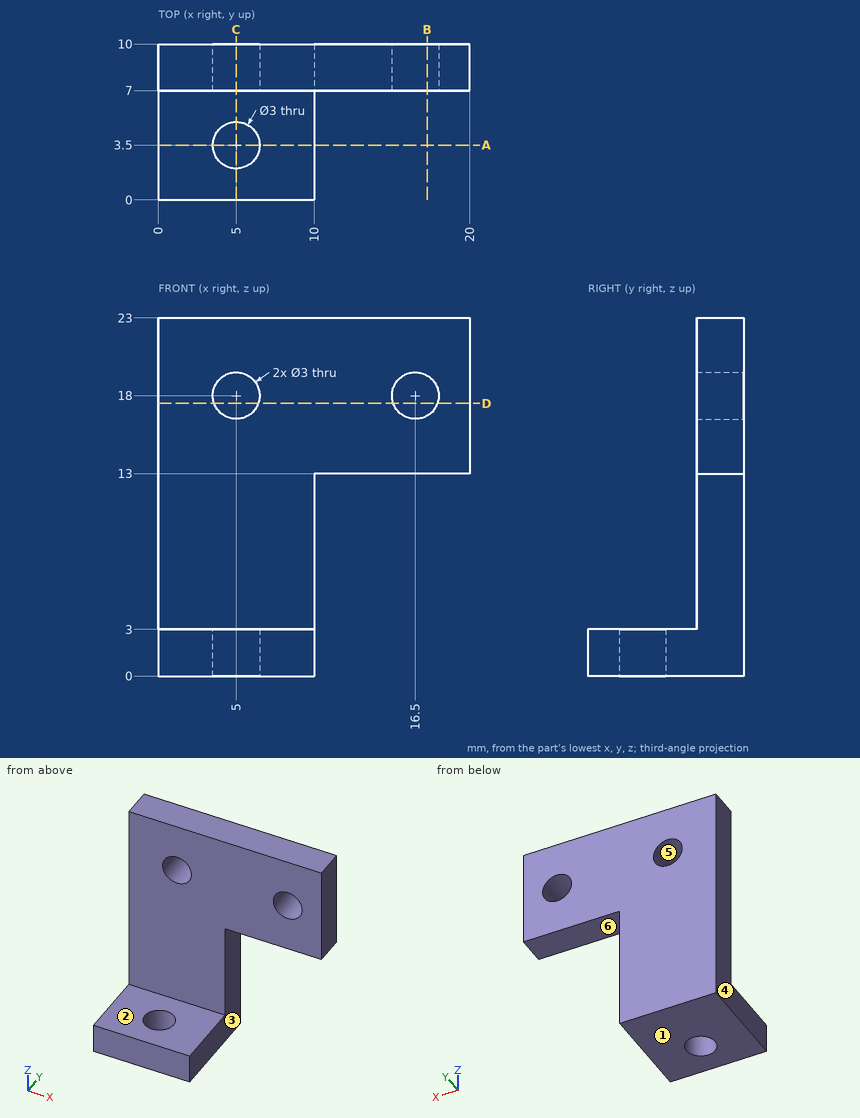
Can you work these out from the drawing? Everything is in mm from the part's minimum corner. A direction names the side the tool comes from. Coordinates: 2 decimals unless noted, no trailing zeros. Loops run counter-clockwise (first coordinate to the right, second up) from the corner with the lowest first, then second, coordinate; pieces in that order, holes last. Notation, with made-up numbers: (43, -30.5) -> (96, -30.5) arc R34 ccw to (96, 3.5) -> close; hole circle Ø3 at (26.5, 15). An arc over 180 degrees is marked (long way). Return JSON: item names as keys, results as strings.
1) If we section it at D-D, the plane z = 17.5: Write out the boundary of the cut face in (x, y).
Results below:
{"outline": "(0, 7) -> (3.59, 7) -> (3.59, 10) -> (0, 10) -> close; (6.41, 7) -> (15.09, 7) -> (15.09, 10) -> (6.41, 10) -> close; (17.91, 7) -> (20, 7) -> (20, 10) -> (17.91, 10) -> close"}
2) Thinking about a two-plate mould opening in Z: for the marked faces 4, 5 and 6, which applies, +Z half, -Z half, draft (parallel to the pull), parting line (faces both ways), or undercut?
Results below:
{"face 4": "draft", "face 5": "undercut", "face 6": "-Z half"}
3) For the marked faces 1, 2 and 3, which set-ups out of +Z, -Z, +X, -X, +Y, -Y let a thin tool reach every point of the face, with its end or its side?
Results below:
{"face 1": "-Z, +X, -X, +Y, -Y", "face 2": "+Z, +X, -X, -Y", "face 3": "-Z, +X, +Y, -Y"}
4) If we section it at A-A, the plane y = 3.5: Write out the boundary of the cut face in (x, z), then the cut area to 3 significant figures.
Results below:
{"outline": "(0, 0) -> (3.5, 0) -> (3.5, 3) -> (0, 3) -> close; (6.5, 0) -> (10, 0) -> (10, 3) -> (6.5, 3) -> close", "area": "21.0 mm²"}
5) Will these pins go through, and if not, where does the flat tip stop? pin 1 (5 mm diameter, centred on x = 6.5, y = 4, fed in from +Z); pin 2 (0.9 mm diameter, centred on x = 13, y = 9, fed in from -Z); pin 3 (4 mm diameter, centred on y = 4.5, z = 6, fed in from -X); pin 4 (8 mm diameter, centred on x = 3.5, z = 18, fed in from -Y).
Results below:
{"pin 1": "z = 3", "pin 2": "z = 13", "pin 3": "through", "pin 4": "y = 7"}
6) If we section it at B-B, the plane x = 17.25: Write out the boundary of the cut face in (y, z).
Results below:
{"outline": "(7, 13) -> (10, 13) -> (10, 16.7) -> (7, 16.7) -> close; (7, 19.3) -> (10, 19.3) -> (10, 23) -> (7, 23) -> close"}
7) If we section it at C-C, the plane x = 5: Write out the boundary of the cut face in (y, z).
Results below:
{"outline": "(0, 0) -> (2, 0) -> (2, 3) -> (0, 3) -> close; (5, 0) -> (10, 0) -> (10, 16.5) -> (7, 16.5) -> (7, 3) -> (5, 3) -> close; (7, 19.5) -> (10, 19.5) -> (10, 23) -> (7, 23) -> close"}
8) I need wall thicknesses on line 1 (X direction, y = 8, z = 18); line 2 (Y direction, x = 5, z = 1.6); line 3 (Y direction, x = 12.25, z = 14.75). Which ranges of each line are inside material? Lowest first, please. Write a range as from..to.
Results below:
{"line 1": "0..3.5, 6.5..15, 18..20", "line 2": "0..2, 5..10", "line 3": "7..10"}
